Here's how the part is built. I have some questions about the finished solid (model axes, mm). Face numbers are marked on the shaded views. A direction names the side the tool comes from. Coordinates: 2 decimals unless noted, no trailing zeros. Loops run counter-clockwise (first coordinate to the right, second up) from the corner with the lowest first, then second, coordinate; pieces in that order, holes last. Notation, with made-up numbers: (-2, 87) -> (52, 87) arc R15 cw to (52, 97) -> close; hole circle Ø4 at (-0.5, 41.5). An arc over 180 degrees is marked (long way). Answer as a JSON object with one key per item and string values. Group by question number.
1) I'm going to push flat-ended pins straight in: pin 1 (5 mm diameter, centred on y = -3, z = 5.5, fed in from +X); pin 2 (2.5 mm diameter, centred on y = -7, z = 4, fed in from +X); pin 3 (4 mm diameter, centred on y = -5, z = 3, fed in from -X). Where does each tip first touch, or does it pass through?
2) If we mould it in two halves opening along X, with no side actions, what happens to the marked faces 6, 7, 8 and 9? For each: +X half, -X half, draft (parallel to the pull), parting line (faces both ways), or undercut.
3) I want a section at B-B (z = 8.15). Write out the boundary of the cut face in (x, y).
4) Which directions (+Z, -Z, +X, -X, +Y, -Y) give clear straight access to the entire face, cutting with the end or side of a thin tool? Please do the marked faces 1, 2, 3, 4 and 5.
5) I need wall thicknesses on probe 1 along X at (y, z) = (-5.15, 8.15); probe 2 along X at (y, z) = (-4.5, 2.75); probe 3 along Z at (x, y) = (5.75, -1.5). Which ranges of each line are inside material? Lowest first, please. Write a range as [from, to].
6) I want a section at A-A (y = -8.5). Count the separate pieces of the cut face and the enclosed holes in it, then the cut area to 3 significant figures.
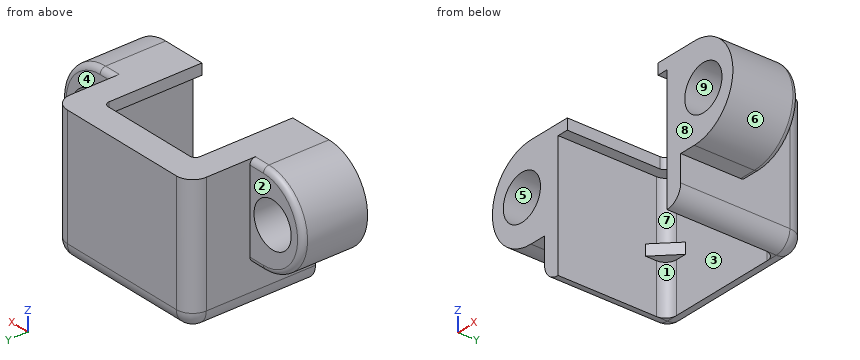
```python
from build123d import *

# Parameters (mm, degrees)
BOSS_EXTRUDE1_DEPTH = 12.4
BOSS_EXTRUDE2_DEPTH = 6
SKETCH4_R           = 2.05
CUT_EXTRUDE1_DEPTH  = 6
FILLET1_R           = 1.5
FILLET2_R           = 0.5
FILLET3_R           = 1
BOSS_EXTRUDE3_DEPTH = 1
FILLET4_R           = 0.5
BOSS_EXTRUDE4_DEPTH = 1
FILLET5_R           = 1.5


with BuildPart() as part:
    # Sketch1 → Boss-Extrude1 (new body)
    with BuildSketch(Plane.XY):
        Polygon((0, 0), (6, 0), (6, -10), (7.5, -10), (7.5, 1.5), (0, 1.5), (-7.5, 1.5), (-7.5, -10), (-6, -10), (-6, 0), align=None)
    extrude(amount=BOSS_EXTRUDE1_DEPTH)

    # Sketch3 → Boss-Extrude2 (add)
    with BuildSketch(Plane.XZ.offset(10)):
        with BuildLine():
            Line((7.5, 3.9), (7.5, 12.4))
            Line((7.5, 12.4), (9, 12.4))
            ThreePointArc((9, 12.4), (13.25, 8.15), (9, 3.9))
            Line((9, 3.9), (7.5, 3.9))
        make_face()
        with BuildLine():
            Line((-7.5, 12.4), (-9, 12.4))
            ThreePointArc((-9, 12.4), (-13.25, 8.15), (-9, 3.9))
            Line((-9, 3.9), (-7.5, 3.9))
            Line((-7.5, 3.9), (-7.5, 12.4))
        make_face()
    extrude(amount=-BOSS_EXTRUDE2_DEPTH)

    # Sketch4 → Cut-Extrude1 (cut)
    with BuildSketch(Plane.XZ.offset(10)):
        with Locations(Location((-10, 8.15, 0), (0, 0, 270))):
            Circle(SKETCH4_R)
        with Locations(Location((10, 8.15, 0), (0, 0, 270))):
            Circle(SKETCH4_R)
    extrude(amount=-CUT_EXTRUDE1_DEPTH, mode=Mode.SUBTRACT)

    # Fillet1
    fillet1_edges = [part.edges().sort_by_distance(p)[0] for p in [
        (-7.5, 1.5, 6.2),
        (7.5, 1.5, 6.2),
    ]]
    fillet(fillet1_edges, radius=FILLET1_R)

    # Fillet2
    fillet2_edges = [part.edges().sort_by_distance(p)[0] for p in [
        (8.25, -4, 3.9),
        (8.25, -4, 12.4),
        (13.25, -4, 8.15),
        (-13.25, -4, 8.15),
        (-8.25, -4, 12.4),
        (-8.25, -4, 3.9),
    ]]
    fillet(fillet2_edges, radius=FILLET2_R)

    # Fillet3
    fillet3_edges = [part.edges().sort_by_distance(p)[0] for p in [
        (6, 0, 6.2),
        (-6, 0, 6.2),
    ]]
    fillet(fillet3_edges, radius=FILLET3_R)

    # Sketch6 → Boss-Extrude3 (add)
    with BuildSketch(Plane(origin=(0, 0, 12.4), x_dir=(-1, 0, 0), z_dir=(0, 0, -1))):
        with BuildLine():
            Line((6, -10), (6, -1))
            ThreePointArc((6, -1), (5.707106781, -0.292893219), (5, 0))
            Line((5, 0), (-5, 0))
            ThreePointArc((-5, 0), (-5.707106781, -0.292893219), (-6, -1))
            Line((-6, -1), (-6, -10))
            Line((-6, -10), (-5, -10))
            Line((-5, -10), (-5, -1))
            Line((-5, -1), (5, -1))
            Line((5, -1), (5, -10))
            Line((5, -10), (6, -10))
        make_face()
    extrude(amount=BOSS_EXTRUDE3_DEPTH)

    # Fillet4
    fillet4_edges = [part.edges().sort_by_distance(p)[0] for p in [
        (5, -1, 11.9),
        (-5, -1, 11.9),
    ]]
    fillet(fillet4_edges, radius=FILLET4_R)

    # Sketch7 → Boss-Extrude4 (add)
    with BuildSketch(Plane(origin=(0, 0, 5.55), x_dir=(-1, 0, 0), z_dir=(0, 0, -1))):
        with BuildLine():
            Line((-4, 0), (-5, 0))
            ThreePointArc((-5, 0), (-5.707106781, -0.292893219), (-6, -1))
            Line((-6, -1), (-6, -2))
            Line((-6, -2), (-4, 0))
        make_face()
        with BuildLine():
            ThreePointArc((5, 0), (5.707106781, -0.292893219), (6, -1))
            Line((6, -1), (6, -2))
            Line((6, -2), (4, 0))
            Line((4, 0), (5, 0))
        make_face()
    extrude(amount=BOSS_EXTRUDE4_DEPTH)

    # Fillet5
    fillet5_edges = [part.edges().sort_by_distance(p)[0] for p in [
        (-7.5, -5, 0),
        (-7.060660172, 1.060660172, 0),
        (0, 1.5, 0),
        (7.060660172, 1.060660172, 0),
        (7.5, -5, 0),
    ]]
    fillet(fillet5_edges, radius=FILLET5_R - 0.0001)  # a hair under: the kernel refuses the full size


solid = part.part
```
Determined:
{
 "1": {"pin 1": "x = 13.2", "pin 2": "x = 12.11", "pin 3": "x = -11.85"},
 "2": {"face 6": "+X half", "face 7": "undercut", "face 8": "draft", "face 9": "undercut"},
 "3": {"outline": "(-13.25, -10) -> (-12.05, -10) -> (-12.05, -4) -> (-12.75, -4) arc R0.5 ccw to (-13.25, -4.5) -> close; (-7.95, -10) -> (-6, -10) -> (-6, -1) arc R1 cw to (-5, 0) -> (5, 0) arc R1 cw to (6, -1) -> (6, -10) -> (7.95, -10) -> (7.95, -4) -> (7.5, -4) -> (7.5, 0) arc R1.5 ccw to (6, 1.5) -> (-6, 1.5) arc R1.5 ccw to (-7.5, 0) -> (-7.5, -4) -> (-7.95, -4) -> close; (12.05, -10) -> (13.25, -10) -> (13.25, -4.5) arc R0.5 ccw to (12.75, -4) -> (12.05, -4) -> close"},
 "4": {"face 1": "-Z, -Y", "face 2": "+Z, -Z, -X, +Y", "face 3": "-Y", "face 4": "+Z, -Z, +X, +Y", "face 5": "+Y, -Y"},
 "5": {"probe 1": "[-13.25, -12.05], [-7.95, -6], [6, 7.95], [12.05, 13.25]", "probe 2": "[-7.5, -6], [6, 7.5]", "probe 3": "[4.55, 5.55], [11.4, 12.4]"},
 "6": {"separate pieces": "2", "enclosed holes": "2", "area": "94.1 mm^2"}
}
